from build123d import *

# Parameters (mm, degrees)
SKETCH2_W           = 22.098
SKETCH2_H           = 19.939
BOSS_EXTRUDE1_DEPTH = 1.5494
BOSS_EXTRUDE3_DEPTH = 1.5494
SKETCH7_R           = 8.1915
BOSS_EXTRUDE4_DEPTH = 12.3952
SKETCH8_R           = 1.5748
SKETCH8_R_2         = 0.4826
CUT_EXTRUDE1_DEPTH  = 2.5494
FILLET1_R           = 0.762


with BuildPart() as part:
    # Sketch2 → Boss-Extrude1 (new body)
    with BuildSketch(Plane(origin=(0, 0, 0), x_dir=(1, 0, 0), z_dir=(0, 1, 0))):
        with Locations((11.049, 9.9695)):
            Rectangle(SKETCH2_W, SKETCH2_H)
    extrude(amount=BOSS_EXTRUDE1_DEPTH)

    # Sketch6 → Boss-Extrude3 (add)
    with BuildSketch(Plane(origin=(0, 1.5494, 0), x_dir=(1, 0, 0), z_dir=(0, 1, 0))):
        with BuildLine():
            ThreePointArc((16.129, 9.017), (14.641102448, 12.609102448), (11.049, 14.097))
            Line((11.049, 14.097), (11.049, 9.017))
            Line((11.049, 9.017), (11.049, 3.937))
            ThreePointArc((11.049, 3.937), (14.641102448, 5.424897552), (16.129, 9.017))
        make_face()
        with BuildLine():
            Line((11.049, 9.017), (11.049, 14.097))
            ThreePointArc((11.049, 14.097), (5.969, 9.017), (11.049, 3.937))
            Line((11.049, 3.937), (11.049, 9.017))
        make_face()
    extrude(amount=BOSS_EXTRUDE3_DEPTH)

    # Sketch7 → Boss-Extrude4 (add)
    with BuildSketch(Plane(origin=(0, 3.0988, 0), x_dir=(1, 0, 0), z_dir=(0, 1, 0))):
        with Locations((11.049, 9.017)):
            Circle(SKETCH7_R)
    extrude(amount=BOSS_EXTRUDE4_DEPTH)

    # Sketch8 → Cut-Extrude1 (cut, through all)
    with BuildSketch(Plane(origin=(0, 1.5494, 0), x_dir=(1, 0, 0), z_dir=(0, 1, 0))):
        with Locations((19.558, 15.494)):
            Circle(SKETCH8_R)
        with Locations((2.54, 2.54)):
            Circle(SKETCH8_R)
        with Locations((16.891, 18.669)):
            Circle(SKETCH8_R_2)
        with Locations((14.351, 18.669)):
            Circle(SKETCH8_R_2)
        with Locations((11.811, 18.669)):
            Circle(SKETCH8_R_2)
        with Locations((9.271, 18.669)):
            Circle(SKETCH8_R_2)
        with Locations((6.731, 18.669)):
            Circle(SKETCH8_R_2)
        with Locations((4.191, 18.669)):
            Circle(SKETCH8_R_2)
        with Locations((1.651, 18.669)):
            Circle(SKETCH8_R_2)
    extrude(amount=-CUT_EXTRUDE1_DEPTH, mode=Mode.SUBTRACT)

    # Fillet1
    fillet1_edges = [part.edges().sort_by_distance(p)[0] for p in [
        (2.8575, 15.494, -9.017),
    ]]
    fillet(fillet1_edges, radius=FILLET1_R)


solid = part.part
Read the model definition and answer for the solid it produces. Units are mm, in the model's axes. A direction names the side the tool comes from. Round coordinates to 2 decimals unless told otherwise and drop trailing zeros. Loops run counter-clockwise (first coordinate to the right, second up) from the corner with the lowest first, then second, coordinate; pieces in that order, holes last. Notation, with made-up numbers: (-15.5, 30) - (32.5, 30) arc R21 ccw to (32.5, 51) - close; hole circle Ø3 at (63.5, 36). An arc over 180 degrees is marked (long way). One line per question, with ' | ' between items. Start each with the question number.
Q1. Flat-ended cylindrical pins translate along their axes: pin 1 (4 mm diameter, centred on x = 2.54, z = -2.54, fed in from +Y); pin 2 (4 mm diameter, centred on x = 16.5, y = 6.5, fed in from -Z); pin 3 (8 mm diameter, centred on y = 10, z = -17.5, fed in from -X). Find the tip coordinate at first contact, or state that the pin passes through.
Q2. Find the intervals of material crossed by L1, parallel to Z at x = 2.54, y = 1.15; L2, parallel to Y at x = 16.75, z = -4.75; L3, parallel to Z at x = 11, y = 8, in increasing order.
Q3. Section B-B on y = 11.75 is taken. Give the vertices of the cut face in (x, z).
Q4. For faces 1 (the flat face through (22.098, 1, -10)), 2 (the flat face through (7, 3.099, -5)), determine the directions among +Z, -Z, +X, -X, +Y, -Y from which every point of the face is accessible in a straight line to the end or side of a thin tool.
Q5. Section A-A on x = 2.54 is taken. Give the vertices of the cut face in (y, z).
Q6. Section C-C on z = -16.75 is taken. Count the separate pieces of the cut face and the enclosed holes in it, plus the area to 3 significant figures.
Q7. Section D-D on x = 20.25 is taken. Give the vertices of the cut face in (y, z).
Q8. For a pull along Z with two mould halves and no side action, classify faces 3 (the cylindrical face through (18.86, 8.83, -11.48)), 4 (the cylindrical face through (3.995, 0.786, -1.937)), 5 (the flat face through (11, 0, -10)) as +Z half, -Z half, draft (parallel to the pull), parting line (faces both ways), or undercut.
Established:
1) pin 1: y = 1.55 | pin 2: z = -16.45 | pin 3: x = 4.19
2) L1: -19.94 to -4.11, -0.97 to 0 | L2: 0 to 1.55, 3.1 to 15.49 | L3: -17.21 to -0.83
3) outline: circle Ø16.38 at (11.05, -9.02)
4) face 1: +Z, -Z, +X, +Y, -Y | face 2: none
5) outline: (0, -19.94) - (1.55, -19.94) - (1.55, -4.11) - (0, -4.11) - close; (0, -0.97) - (1.55, -0.97) - (1.55, 0) - (0, 0) - close
6) separate pieces: 3 | enclosed holes: 0 | area: 97.3 mm²
7) outline: (0, -19.94) - (1.55, -19.94) - (1.55, -16.91) - (0, -16.91) - close; (0, -14.08) - (1.55, -14.08) - (1.55, 0) - (0, 0) - close
8) face 3: parting line | face 4: undercut | face 5: draft
